Input: dimensioned drawing with shaded views. Units: mm. Origin: part minimum x, y, z. Give positions to 0.01 mm unless a question says otherwise; leave off trailing zeros. Write each loop counter-clockwise with the first axis right and the second up, starting at its lowest first coordinate (ties: lowest second). Pieces come first, ordered by that corner, then holes. Notation, with made-up numbers: (15.5, 69) -> (42.5, 69) arc R20 ccw to (42.5, 102) -> close; hole circle Ø10 at (33, 67.25). An arc over 180 degrees is marked (long way). Answer as a JSON object with one key per item and string values. Group by question number.
(1) Section query B-B on x = 2.5. Output: boundary loops of the cut face in (y, z), plus the area to 4 significant figures.
(2) Contact query for a flat-ended pin moving along its axis: pin 1 Ø1.9 at (x, y) = (43.2, 18.8) entering from -Z. Output: stop coordinate, or through.
(3) Section query A-A on y = 2.5. Output: boundary loops of the cut face in (x, z).
(4) Material intervals for probe 1 along Y at (x, z) = (2.5, 1.2); probe 2 along X at (y, z) = (18.8, 0.8); probe 3 along X at (y, z) = (2.5, 1.3), sorted ascending.
(5) Section query C-C on z = 0.8. Output: boundary loops of the cut face in (x, y), plus the area to 3 significant figures.
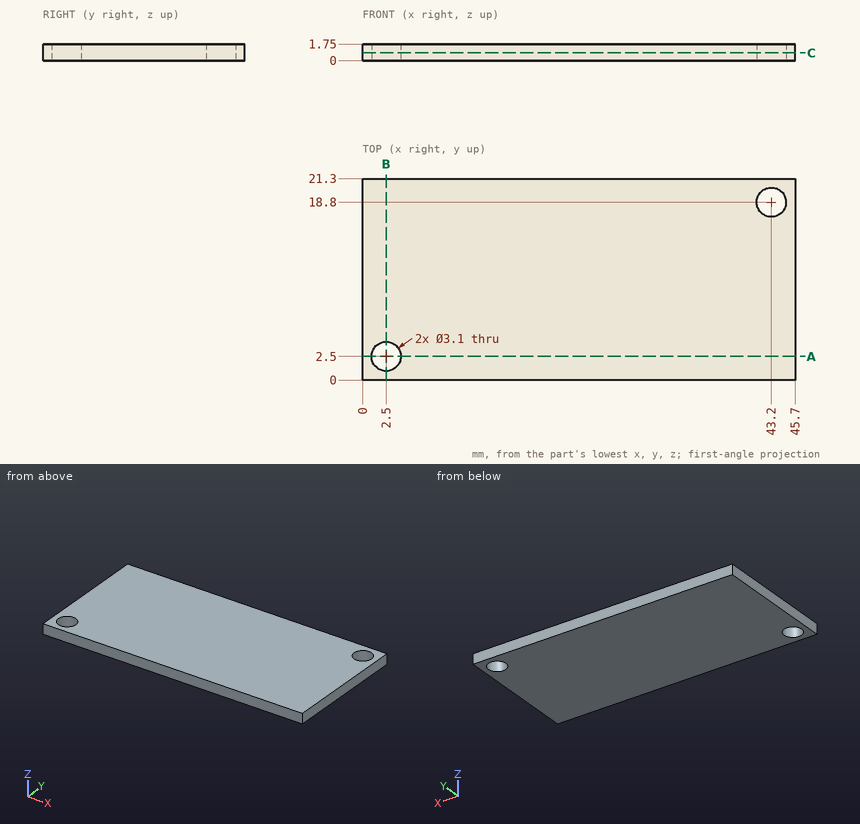
Answer list:
{
 "1": {"outline": "(0, 0) -> (0.95, 0) -> (0.95, 1.75) -> (0, 1.75) -> close; (4.05, 0) -> (21.3, 0) -> (21.3, 1.75) -> (4.05, 1.75) -> close", "area": "31.85 mm2"},
 "2": {"pin 1": "through"},
 "3": {"outline": "(0, 0) -> (0.95, 0) -> (0.95, 1.75) -> (0, 1.75) -> close; (4.05, 0) -> (45.7, 0) -> (45.7, 1.75) -> (4.05, 1.75) -> close"},
 "4": {"probe 1": "0 to 0.95, 4.05 to 21.3", "probe 2": "0 to 41.65, 44.75 to 45.7", "probe 3": "0 to 0.95, 4.05 to 45.7"},
 "5": {"outline": "(0, 0) -> (45.7, 0) -> (45.7, 21.3) -> (0, 21.3) -> close; hole circle Ø3.1 at (2.5, 2.5); hole circle Ø3.1 at (43.2, 18.8)", "area": "958 mm2"}
}
